The model under review builds one solid part; all positions refer to its coordinate system, in mm. Round coordinates to 2 decimals unless told otherwise and drop trailing zeros.
```python
from build123d import *

# Parameters (mm, degrees)
BOSS_EXTRUDE1_DEPTH   = 2.5
SKETCH24_R            = 3.9
CUT_EXTRUDE2_DEPTH    = 307.16304509
SKETCH1_R             = 12
SKETCH1_R_2           = 15
CUT_EXTRUDE3_DEPTH    = 307.16304509
SKETCH4_W             = 19.05
SKETCH4_H             = 19.05
CUT_EXTRUDE5_DEPTH    = 326.800182738
CUT_EXTRUDE6_DEPTH    = 307.16304509
F_3_0MM_DOWEL_HOLE1_D = 3
FILLET1_R             = 1
CHAMFER1_SIZE         = 1
CHAMFER2_SIZE         = 0.5


with BuildPart() as part:
    # Sketch2 → Boss-Extrude1 (new body)
    with BuildSketch(Plane.XY):
        with BuildLine():
            Line((8.41186441, 15.286374556), (8.41186441, 109.410267401))
            Line((8.41186441, 109.410267401), (6.41186441, 107.410267401))
            Line((6.41186441, 107.410267401), (6.41186441, 15.286374556))
            ThreePointArc((6.41186441, 15.286374556), (9.340796598, 8.215306744), (16.41186441, 5.286374556))
            Line((16.41186441, 5.286374556), (264.168886442, 5.286374556))
            ThreePointArc((264.168886442, 5.286374556), (271.239954254, 8.215306744), (274.168886442, 15.286374556))
            Line((274.168886442, 15.286374556), (274.168886442, 107.410267401))
            Line((274.168886442, 107.410267401), (272.168886442, 109.410267401))
            Line((272.168886442, 109.410267401), (272.168886442, 15.286374556))
            ThreePointArc((272.168886442, 15.286374556), (269.825740692, 9.629520306), (264.168886442, 7.286374556))
            Line((264.168886442, 7.286374556), (16.41186441, 7.286374556))
            ThreePointArc((16.41186441, 7.286374556), (10.755010161, 9.629520306), (8.41186441, 15.286374556))
        make_face()
        with BuildLine():
            Line((247.340459317, 134.238694526), (33.240291535, 134.238694526))
            Line((33.240291535, 134.238694526), (8.41186441, 109.410267401))
            Line((8.41186441, 109.410267401), (8.41186441, 15.286374556))
            ThreePointArc((8.41186441, 15.286374556), (10.755010161, 9.629520306), (16.41186441, 7.286374556))
            Line((16.41186441, 7.286374556), (264.168886442, 7.286374556))
            ThreePointArc((264.168886442, 7.286374556), (269.825740692, 9.629520306), (272.168886442, 15.286374556))
            Line((272.168886442, 15.286374556), (272.168886442, 109.410267401))
            Line((272.168886442, 109.410267401), (247.340459317, 134.238694526))
        make_face()
        Polygon((33.240291535, 134.238694526), (30.41186441, 134.238694526), (8.41186441, 112.238694526), (8.41186441, 109.410267401), align=None)
        Polygon((8.41186441, 109.410267401), (8.41186441, 112.238694526), (6.41186441, 110.238694526), (6.41186441, 107.410267401), align=None)
        Polygon((32.41186441, 136.238694526), (30.41186441, 134.238694526), (33.240291535, 134.238694526), (35.240291535, 136.238694526), align=None)
        Polygon((35.240291535, 136.238694526), (33.240291535, 134.238694526), (247.340459317, 134.238694526), (245.340459317, 136.238694526), align=None)
        Polygon((272.168886442, 112.238694526), (272.168886442, 109.410267401), (274.168886442, 107.410267401), (274.168886442, 110.238694526), align=None)
        Polygon((250.168886442, 134.238694526), (247.340459317, 134.238694526), (272.168886442, 109.410267401), (272.168886442, 112.238694526), align=None)
        Polygon((245.340459317, 136.238694526), (247.340459317, 134.238694526), (250.168886442, 134.238694526), (248.168886442, 136.238694526), align=None)
    extrude(amount=-BOSS_EXTRUDE1_DEPTH)

    # Sketch24 → Cut-Extrude2 (cut, through all)
    with BuildSketch(Plane.XY):
        with Locations((37.41186441, 124.238694526)):
            Circle(SKETCH24_R)
        with Locations((50.91186441, 124.238694526)):
            Circle(SKETCH24_R)
        with Locations((64.41186441, 124.238694526)):
            Circle(SKETCH24_R)
        with Locations((216.168886442, 124.238694526)):
            Circle(SKETCH24_R)
        with Locations((229.668886442, 124.238694526)):
            Circle(SKETCH24_R)
        with Locations((243.168886442, 124.238694526)):
            Circle(SKETCH24_R)
        with BuildLine():
            Line((193.298949614, 125.738694526), (193.298949614, 122.738694526))
            ThreePointArc((193.298949614, 122.738694526), (194.798949614, 121.238694526), (196.298949614, 122.738694526))
            Line((196.298949614, 122.738694526), (196.298949614, 125.738694526))
            ThreePointArc((196.298949614, 125.738694526), (194.798949614, 127.238694526), (193.298949614, 125.738694526))
        make_face()
    extrude(amount=-CUT_EXTRUDE2_DEPTH, mode=Mode.SUBTRACT)

    # Sketch1 → Cut-Extrude3 (cut, through all)
    with BuildSketch(Plane.XY):
        with Locations((24.41186441, 82.179064133)):
            Circle(SKETCH1_R)
        with Locations((168.091946024, 58.360067852)):
            Circle(SKETCH1_R)
        with Locations((194.873540874, 70.729230202)):
            Circle(SKETCH1_R)
        with Locations((224.358659158, 69.792320505)):
            Circle(SKETCH1_R)
        with Locations((253.510608286, 65.274150291)):
            Circle(SKETCH1_R)
        with Locations((256.168886442, 94.654135948)):
            Circle(SKETCH1_R)
        with Locations((227.016937315, 99.172306162)):
            Circle(SKETCH1_R)
        with Locations((197.531819031, 100.10921586)):
            Circle(SKETCH1_R)
        with Locations((170.75022418, 87.740053509)):
            Circle(SKETCH1_R)
        with Locations((191.774681199, 29.091460603)):
            Circle(SKETCH1_R_2)
        with Locations((157.891946024, 26.270067852)):
            Circle(SKETCH1_R_2)
        with Locations((123.891946024, 26.270067852)):
            Circle(SKETCH1_R_2)
        with Locations((90.009210849, 29.091460603)):
            Circle(SKETCH1_R_2)
        with Locations((173.429012786, 117.118176179)):
            Circle(SKETCH1_R)
    extrude(amount=-CUT_EXTRUDE3_DEPTH, mode=Mode.SUBTRACT)

    # Sketch4 → Cut-Extrude5 (cut, through all)
    with BuildSketch(Plane(origin=(-30.20834345, 20.07496957, 0), x_dir=(0.9781476007338056, -0.2079116908177598, 0), z_dir=(0, 0, 1))):
        with Locations((95.695570415, 103.716725336)):
            Rectangle(SKETCH4_W, SKETCH4_H)
        Polygon((124.270570415, 94.191725336), (105.220570415, 94.191725336), (105.220570415, 84.497139957), (124.270570415, 84.157969199), align=None)
        Polygon((105.220570415, 84.497139957), (105.220570415, 75.141725336), (124.270570415, 75.141725336), (124.270570415, 84.157969199), align=None)
        Polygon((105.220570415, 75.141725336), (95.695570415, 84.666725336), (86.170570415, 84.836310715), (86.170570415, 75.141725336), align=None)
        Polygon((105.220570415, 84.497139957), (95.695570415, 84.666725336), (105.220570415, 75.141725336), align=None)
        Polygon((105.220570415, 94.191725336), (86.170570415, 94.191725336), (95.695570415, 84.666725336), (105.220570415, 84.497139957), align=None)
        Polygon((95.695570415, 84.666725336), (86.170570415, 94.191725336), (86.170570415, 84.836310715), align=None)
        Polygon((86.170570415, 75.141725336), (86.170570415, 84.836310715), (67.120570415, 85.175481473), (67.120570415, 75.141725336), align=None)
        Polygon((86.170570415, 84.836310715), (86.170570415, 94.191725336), (67.120570415, 94.191725336), (67.120570415, 85.175481473), align=None)
    extrude(amount=-CUT_EXTRUDE5_DEPTH, mode=Mode.SUBTRACT)

    # Sketch27 → Cut-Extrude6 (cut, through all)
    with BuildSketch(Plane.XY):
        with BuildLine():
            Line((54.735010804, 96.86991883), (56.41235194, 97.9591969))
            ThreePointArc((56.41235194, 97.9591969), (55.029042337, 98.253228433), (54.735010804, 96.86991883))
        make_face()
        with BuildLine():
            Line((51.36235616, 81.002826242), (52.45163423, 79.325485106))
            ThreePointArc((52.45163423, 79.325485106), (51.068324627, 79.619516639), (51.36235616, 81.002826242))
        make_face()
        with BuildLine():
            Line((105.586150406, 68.031395041), (107.263491542, 69.120673111))
            ThreePointArc((107.263491542, 69.120673111), (106.969460009, 67.737363508), (105.586150406, 68.031395041))
        make_face()
        with BuildLine():
            Line((109.546868116, 86.665106835), (110.636146186, 84.987765699))
            ThreePointArc((110.636146186, 84.987765699), (110.930177719, 86.371075302), (109.546868116, 86.665106835))
        make_face()
        with BuildLine():
            Line((77.329440308, 111.542912914), (79.006781444, 112.632190984))
            ThreePointArc((79.006781444, 112.632190984), (77.623471841, 112.926222516), (77.329440308, 111.542912914))
        make_face()
        with BuildLine():
            Line((94.873874032, 109.259536339), (95.963152102, 107.582195203))
            ThreePointArc((95.963152102, 107.582195203), (96.257183635, 108.965504806), (94.873874032, 109.259536339))
        make_face()
    extrude(amount=-CUT_EXTRUDE6_DEPTH, mode=Mode.SUBTRACT)

    # 3.0mm Dowel Hole1 (through all)
    with Locations(Plane.XY):
        with Locations((25.42227205, 117.228286886), (16.41186441, 15.286374556), (264.168886442, 15.286374556), (255.158478802, 117.228286886)):
            Hole(F_3_0MM_DOWEL_HOLE1_D / 2)

    # Fillet1
    fillet1_edges = [part.edges().sort_by_distance(p)[0] for p in [
        (73.662754131, 94.292510723, -1.25),
        (92.296465925, 90.331793012, -1.25),
        (77.329440308, 111.542912914, -1.25),
        (79.006781444, 112.632190984, -1.25),
        (94.873874032, 109.259536339, -1.25),
        (95.963152102, 107.582195203, -1.25),
        (109.546868116, 86.665106835, -1.25),
        (110.636146186, 84.987765699, -1.25),
        (107.263491542, 69.120673111, -1.25),
        (105.586150406, 68.031395041, -1.25),
        (52.45163423, 79.325485106, -1.25),
        (51.36235616, 81.002826242, -1.25),
        (54.735010804, 96.86991883, -1.25),
        (56.41235194, 97.9591969, -1.25),
    ]]
    fillet(fillet1_edges, radius=FILLET1_R)

    # Chamfer1
    chamfer1_edges = [part.edges().sort_by_distance(p)[0] for p in [
        (274.168886442, 62.762534541, 0),
        (271.239954254, 8.215306744, 0),
        (140.290375426, 5.286374556, 0),
        (9.340796598, 8.215306744, 0),
        (6.41186441, 62.762534541, 0),
        (19.41186441, 123.238694526, 0),
        (140.290375426, 136.238694526, 0),
        (261.168886442, 123.238694526, 0),
    ]]
    chamfer(chamfer1_edges, length=CHAMFER1_SIZE)

    # Chamfer2
    chamfer2_edges = [part.edges().sort_by_distance(p)[0] for p in [
        (12.41186441, 82.179064133, 0),
        (244.168886442, 94.654135948, 0),
        (215.016937315, 99.172306162, 0),
        (185.531819031, 100.10921586, 0),
        (158.75022418, 87.740053509, 0),
        (161.429012786, 117.118176179, 0),
        (241.510608286, 65.274150291, 0),
        (212.358659158, 69.792320505, 0),
        (182.873540874, 70.729230202, 0),
        (156.091946024, 58.360067852, 0),
        (176.774681199, 29.091460603, 0),
        (142.891946024, 26.270067852, 0),
        (108.891946024, 26.270067852, 0),
        (75.009210849, 29.091460603, 0),
        (106.969460009, 67.737363508, 0),
        (77.623471841, 112.926222516, 0),
        (86.940327738, 110.945863661, 0),
        (96.257183635, 108.965504806, 0),
        (94.198949632, 99.282275143, 0),
        (101.246948056, 88.429309305, 0),
        (110.930177719, 86.371075302, 0),
        (108.949818864, 77.054219405, 0),
        (79.018892318, 73.678440073, 0),
        (51.068324627, 79.619516639, 0),
        (53.048683482, 88.936372536, 0),
        (55.029042337, 98.253228433, 0),
        (64.712272, 96.19499443, 0),
        (75.565237838, 103.242992853, 0),
        (56.483009318, 97.982319264, 0),
        (54.685148528, 96.814774815, 0),
        (51.339233796, 81.07348362, 0),
        (52.506778244, 79.27562283, 0),
        (73.437157256, 94.639899446, 0),
        (79.077438822, 112.655313348, 0),
        (77.279578032, 111.487768899, 0),
        (94.818730018, 109.309398615, 0),
        (95.986274466, 107.511537825, 0),
        (92.643854649, 90.557389887, 0),
        (109.491724102, 86.714969111, 0),
        (110.65926855, 84.917108321, 0),
        (107.313353817, 69.175817126, 0),
        (105.515493027, 68.008272677, 0),
        (33.51186441, 124.238694526, 0),
        (194.798949614, 127.238694526, 0),
        (193.298949614, 124.238694526, 0),
        (194.798949614, 121.238694526, 0),
        (196.298949614, 124.238694526, 0),
        (239.268886442, 124.238694526, 0),
        (225.768886442, 124.238694526, 0),
        (212.268886442, 124.238694526, 0),
        (60.51186441, 124.238694526, 0),
        (47.01186441, 124.238694526, 0),
    ]]
    chamfer(chamfer2_edges, length=CHAMFER2_SIZE)


solid = part.part
```
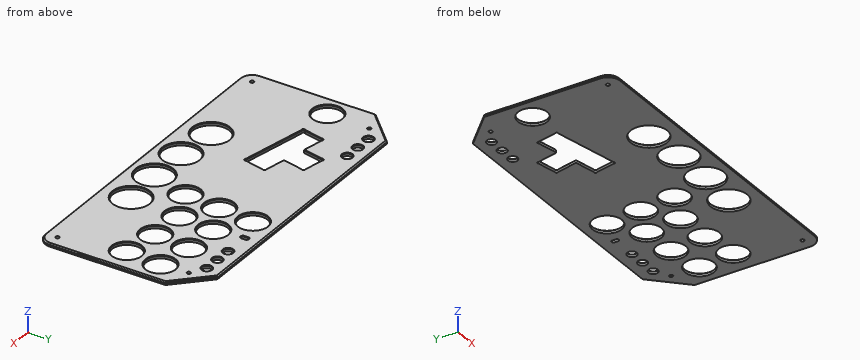
(1) Insertion check: pin 1 (7 mm diameter, centred on x = 243.17, y = 124.24, fed in from -Z); pin 2 (0.6 mm diameter, centred on y = 123.5, z = -1.5, fed in from +X). Each pin has a flat end and moves straight along its axis. Give the tip position at first contact, or say it passes through.
Data:
pin 1: passes through
pin 2: stops at x = 261.21
(2) Consider section A-A (z = -1.85). State how many separate pieces and enclosed holes the cut face has, and give its area (3 significant figures).
Data:
separate pieces: 1
enclosed holes: 26
area: 25,200 mm2
(3) To check wall thickness, follow probe 1 along Y at (x, z) = (90.5, -1.6); probe 2 along X at (y, z) = (55, -0.6); probe 3 along X at (y, z) = (34, -1.05). State the ranges of each line that lie inside material, in increasing order.
Data:
probe 1: y = 5.29 to 14.1, 44.08 to 71.24, 110.19 to 136.24
probe 2: x = 6.81 to 156.57, 179.61 to 247.31, 259.71 to 273.77
probe 3: x = 6.41 to 75.84, 104.18 to 111.04, 136.75 to 145.04, 170.75 to 177.6, 205.95 to 274.17
